```python
from build123d import *

# Parameters (mm, degrees)
ESQUISSE1_W             = 35
ESQUISSE1_H             = 13
ESQUISSE1_R             = 1.75
ESQUISSE1_R_2           = 1.5
BOSS_EXTRU_1_DEPTH      = 5
ESQUISSE2_W             = 35
ESQUISSE2_H             = 13
ESQUISSE2_R             = 1.5
ESQUISSE2_R_2           = 1.75
ESQUISSE2_W_2           = 15
ESQUISSE2_H_2           = 8
BOSS_EXTRU_2_DEPTH      = 15
ESQUISSE3_W             = 35
ESQUISSE3_H             = 13
ESQUISSE3_R             = 3
BOSS_EXTRU_3_DEPTH      = 2
ESQUISSE9_R             = 1.75
ENL_V_MAT_EXTRU_5_DEPTH = 31.971761332
ESQUISSE5_W             = 52.735375718
ESQUISSE5_H             = 32.07387294
ENL_V_MAT_EXTRU_1_DEPTH = 31.008332211
ENL_V_MAT_EXTRU_2_DEPTH = 28.358728137
ESQUISSE4_W             = 5.5
ESQUISSE4_H             = 2.5
ENL_V_MAT_EXTRU_3_DEPTH = 4
ENL_V_MAT_EXTRU_4_DEPTH = 2.5
ENL_V_MAT_EXTRU_6_DEPTH = 2.5


with BuildPart() as part:
    # Esquisse1 → Boss.-Extru.1 (new body)
    with BuildSketch(Plane(origin=(0, 0, 0), x_dir=(1, 0, 0), z_dir=(0, 1, 0))):
        Rectangle(ESQUISSE1_W, ESQUISSE1_H)
        with Locations(Location((-12.5, 0, 0), (0, 0, 270))):
            Circle(ESQUISSE1_R, mode=Mode.SUBTRACT)
        with Locations(Location((12.5, 0, 0), (0, 0, 270))):
            Circle(ESQUISSE1_R_2, mode=Mode.SUBTRACT)
        Polygon((-10.5, -6), (10.5, -6), (9, 6), (-9, 6), align=None, mode=Mode.SUBTRACT)
    extrude(amount=BOSS_EXTRU_1_DEPTH)

    # Esquisse2 → Boss.-Extru.2 (add)
    with BuildSketch(Plane(origin=(0, 5, 0), x_dir=(1, 0, 0), z_dir=(0, 1, 0))):
        Rectangle(ESQUISSE2_W, ESQUISSE2_H)
        with Locations(Location((12.5, 0, 0), (0, 0, 270))):
            Circle(ESQUISSE2_R, mode=Mode.SUBTRACT)
        with Locations(Location((-12.5, 0, 0), (0, 0, 270))):
            Circle(ESQUISSE2_R_2, mode=Mode.SUBTRACT)
        Rectangle(ESQUISSE2_W_2, ESQUISSE2_H_2, mode=Mode.SUBTRACT)
    extrude(amount=BOSS_EXTRU_2_DEPTH)

    # Esquisse3 → Boss.-Extru.3 (add)
    with BuildSketch(Plane(origin=(0, 20, 0), x_dir=(1, 0, 0), z_dir=(0, 1, 0))):
        Rectangle(ESQUISSE3_W, ESQUISSE3_H)
        with Locations(Location((0, 0, 0), (0, 0, 270))):
            Circle(ESQUISSE3_R, mode=Mode.SUBTRACT)
    extrude(amount=BOSS_EXTRU_3_DEPTH)

    # Esquisse9 → Enlèv. mat.-Extru.5 (cut, through all)
    with BuildSketch(Plane.XY.offset(6.5)):
        with Locations((-13, 17)):
            Circle(ESQUISSE9_R)
        with Locations((13, 17)):
            Circle(ESQUISSE9_R)
    extrude(amount=-ENL_V_MAT_EXTRU_5_DEPTH, mode=Mode.SUBTRACT)

    # Esquisse5 → Enlèv. mat.-Extru.1 (cut, through all)
    with BuildSketch(Plane(origin=(0, 0, 4), x_dir=(-1, 0, 0), z_dir=(0, 0, -1))):
        with Locations((3.176053458, 10.251854402)):
            Rectangle(ESQUISSE5_W, ESQUISSE5_H)
    extrude(amount=-ENL_V_MAT_EXTRU_1_DEPTH, mode=Mode.SUBTRACT)

    # Esquisse6 → Enlèv. mat.-Extru.2 (cut, through all)
    with BuildSketch(Plane.XZ.offset(-20)):
        with BuildLine():
            Line((-3, 4), (-3, 0))
            ThreePointArc((-3, 0), (0, 3), (3, 0))
            Line((3, 0), (3, 4))
            Line((3, 4), (-3, 4))
        make_face()
    extrude(amount=-ENL_V_MAT_EXTRU_2_DEPTH, mode=Mode.SUBTRACT)

    # Esquisse4 → Enlèv. mat.-Extru.3 (cut)
    with BuildSketch(Plane(origin=(0, 0, 4), x_dir=(-1, 0, 0), z_dir=(0, 0, -1))):
        with Locations((12.5, 8)):
            Rectangle(ESQUISSE4_W, ESQUISSE4_H)
    enl_v_mat_extru_3 = extrude(amount=ENL_V_MAT_EXTRU_3_DEPTH, mode=Mode.SUBTRACT)

    # Esquisse7 → Enlèv. mat.-Extru.4 (cut)
    with BuildSketch(Plane(origin=(0, 6.75, 0), x_dir=(1, 0, 0), z_dir=(0, 1, 0))):
        Polygon((-9.75, -1.58771324), (-9.75, 1.58771324), (-12.5, 3.175426481), (-15.25, 1.58771324), (-15.25, -1.58771324), (-12.5, -3.175426481), align=None)
    enl_v_mat_extru_4 = extrude(amount=ENL_V_MAT_EXTRU_4_DEPTH, mode=Mode.SUBTRACT)

    # Symétrie1: Enlèv. mat.-Extru.3, Enlèv. mat.-Extru.4 across plane
    add(enl_v_mat_extru_3.mirror(Plane.ZY), mode=Mode.SUBTRACT)
    add(enl_v_mat_extru_4.mirror(Plane.ZY), mode=Mode.SUBTRACT)

    # Esquisse10 → Enlèv. mat.-Extru.6 (cut)
    with BuildSketch(Plane(origin=(0, 0, -6.5), x_dir=(-1, 0, 0), z_dir=(0, 0, -1))):
        Polygon((-10.25, 15.41228676), (-10.25, 18.58771324), (-13, 20.175426481), (-15.75, 18.58771324), (-15.75, 15.41228676), (-13, 13.824573519), align=None)
        Polygon((13, 13.824573519), (15.75, 15.41228676), (15.75, 18.58771324), (13, 20.175426481), (10.25, 18.58771324), (10.25, 15.41228676), align=None)
    extrude(amount=-ENL_V_MAT_EXTRU_6_DEPTH, mode=Mode.SUBTRACT)


solid = part.part
```
Check sheet for the modelled part. Datum: model origin and axes. Units: mm. A direction names the side the tool comes from. Round coordinates to 2 decimals unless told otherwise and drop trailing zeros. Loops run counter-clockwise (first coordinate to the right, second up) from the corner with the lowest first, then second, coordinate; pieces in that order, holes last. Notation, with made-up numbers: (-39.75, -17.75) -> (-22.75, -17.75) arc R16 ccw to (-22.75, 5.25) -> close; hole circle Ø10 at (-37.75, 72). An arc over 180 degrees is marked (long way). Write item = value, one per line. Start each with the question number.
1) Sectioned sample at C-C, the plane y = 10. Record the cut outline in (x, z).
2) Sectioned sample at D-D, the plane y = 19.5. Record the cut outline in (x, z).
3) Sectioned sample at B-B, the plane z = -5.5. Record the cut outline in (x, y).
4) Release check for a two-part mould opening along Z. For faces 5 (the cylindrical face through (0, 21, -3)), 6 (the flat face through (-11.7, 15.6, -4)), 7 (the cylindrical face through (-10.765, 13.355, -0.228)) record: released by +Z, released by -Z, zero draft, split by the parting line, or undercut.
5) Thickness scan on probe 1 along Y at (x, z) = (13, 2.25); probe 2 along Z at (x, y) = (12.5, 14.5); probe 3 along X at (y, z) = (17.25, 0). Record the ranges inside material, lowest first.
6) Sectioned sample at A-A, the plane y = 4. Record the cut outline in (x, z), plus the area to 3 significant figures.
7) Set-up check for faces 1 (the flat face through (12, 20, 0)), 2 (the flat face through (12, 9.25, 2)), 3 (the flat face through (-2, 20, -3)), 4 (the flat face through (-11.606, 14.63, -5.268)): record each of +Z, -Z, +X, -X, +Y, -Y from which the full face is reachable in a straight line by a thin tool's end or side.
8) Gauge pin test, flat ends, axial feed: pin 1 Ø1.5 at (x, y) = (-3, 3) entering from +Z; pin 2 Ø2.5 at (x, z) = (-3, -0.5) entering from -Y; pin 3 Ø5 at (x, z) = (-1.5, -2) entering from -Y. Record the tip position at first contact, or that the pin passes through.
Results are:
q1.outline = (-17.5, -6.5) -> (17.5, -6.5) -> (17.5, 4) -> (7.5, 4) -> (7.5, -4) -> (-7.5, -4) -> (-7.5, 4) -> (-17.5, 4) -> close; hole circle Ø3.5 at (-12.5, 0); hole circle Ø3 at (12.5, 0)
q2.outline = (-17.5, -6.5) -> (-14.17, -6.5) -> (-14.17, -4) -> (-11.83, -4) -> (-11.83, -6.5) -> (11.83, -6.5) -> (11.83, -4) -> (14.17, -4) -> (14.17, -6.5) -> (17.5, -6.5) -> (17.5, 4) -> (7.5, 4) -> (7.5, -4) -> (-7.5, -4) -> (-7.5, 4) -> (-17.5, 4) -> close; hole circle Ø3.5 at (-12.5, 0); hole circle Ø3 at (12.5, 0)
q3.outline = (-17.5, 0) -> (-9.06, 0) -> (-9.06, 5) -> (9.06, 5) -> (9.06, 0) -> (17.5, 0) -> (17.5, 22) -> (-17.5, 22) -> close; hole (-15.75, 15.41) -> (-13, 13.82) -> (-10.25, 15.41) -> (-10.25, 18.59) -> (-13, 20.18) -> (-15.75, 18.59) -> close; hole (10.25, 15.41) -> (13, 13.82) -> (15.75, 15.41) -> (15.75, 18.59) -> (13, 20.18) -> (10.25, 18.59) -> close
q4.face_5 = released by +Z
q4.face_6 = released by -Z
q4.face_7 = undercut
q5.probe_1 = 0 to 6.75, 9.25 to 15.25, 18.75 to 22
q5.probe_2 = -4 to -1.5, 1.5 to 4
q5.probe_3 = -17.5 to -14.73, -10.75 to -7.5, 7.5 to 11, 14.73 to 17.5
q6.outline = (-17.5, -6.5) -> (17.5, -6.5) -> (17.5, 4) -> (10.25, 4) -> (9, -6) -> (-9, -6) -> (-10.25, 4) -> (-17.5, 4) -> close; hole circle Ø3.5 at (-12.5, 0); hole circle Ø3 at (12.5, 0)
q6.area = 158 mm^2
q7.face_1 = -Y
q7.face_2 = +Z
q7.face_3 = +Z, -Y
q7.face_4 = -Z
q8.pin_1 = -6
q8.pin_2 = 20
q8.pin_3 = 5
